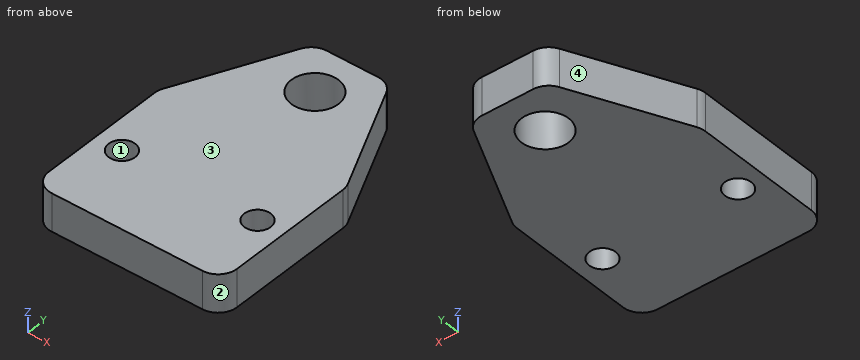
```python
from build123d import *

# Parameters (mm, degrees)
BOSS_EXTRU_1_DEPTH           = 10
ENL_V_MAT_EXTRU_1_DEPTH      = 77.870020164
ENL_V_MAT_EXTRU_1_DEPTH_BACK = 77.870020164
ESQUISSE2_R                  = 3.5
CONG_1_R                     = 5
ESQUISSE3_R                  = 6.25
ENL_V_MAT_EXTRU_2_DEPTH      = 77.870020164


with BuildPart() as part:
    # Esquisse1 → Boss.-Extru.1 (new body)
    with BuildSketch(Plane.XY):
        Polygon((-25, 0), (25, 0), (25, 40), (10, 72), (-10, 72), (-25, 40), align=None)
    extrude(amount=BOSS_EXTRU_1_DEPTH)

    # Esquisse2 → Enlèv. mat.-Extru.1 (cut, two sides: drawn at the far end of the back side and taken through both)
    with BuildSketch(Plane.XY.offset(10).offset(-ENL_V_MAT_EXTRU_1_DEPTH_BACK)):
        with Locations((18, 20)):
            Circle(ESQUISSE2_R)
        with Locations((-18, 20)):
            Circle(ESQUISSE2_R)
    extrude(amount=ENL_V_MAT_EXTRU_1_DEPTH + ENL_V_MAT_EXTRU_1_DEPTH_BACK, mode=Mode.SUBTRACT)

    # Congé1
    cong_1_edges = [part.edges().sort_by_distance(p)[0] for p in [
        (25, 0, 5),
        (-25, 0, 5),
        (-25, 40, 5),
        (-10, 72, 5),
        (10, 72, 5),
        (25, 40, 5),
    ]]
    fillet(cong_1_edges, radius=CONG_1_R)

    # Esquisse3 → Enlèv. mat.-Extru.2 (cut, through all)
    with BuildSketch(Plane.XY.offset(10)):
        with Locations((0, 60)):
            Circle(ESQUISSE3_R)
    extrude(amount=-ENL_V_MAT_EXTRU_2_DEPTH, mode=Mode.SUBTRACT)


solid = part.part
```
Geometry check sheet. Reference: the model listing, model coordinates, mm. Face numbers are marked on the shaded views. Give positions to 0.01 mm unless a question says otherwise; leave off trailing zeros. Order: outer loops, then holes, each group sorted by start corner. A loop starts at its lowest first (then second) coordinate and runs counter-clockwise, first axis right, second up. Notation, with made-up numbers: (-33, 24) -> (26, 24) arc R18 ccw to (26, 30) -> close; hole circle Ø4 at (34, -17.5). An arc over 180 degrees is marked (long way). Write each question's results on one line, items separated by ' | '. Start each with the question number.
(1) Mould release check, pull along X, two halves, no side actions. Record for the marked faces 1, 2, 3 and 4: pulls with the +X half, pulls with the -X half, needs draft (parallel to the pull), parting line crosses it, or undercut.
(2) Scan lines: line 1 (X direction, y = 20, z = 5.5); line 2 (Y direction, x = 0, z = 3); line 3 (X direction, y = 22, z = 9.5). Record each from-to range of solid material in increasing order.
(3) Sectioned sample at D-D (y = 57.5). Enter the section's corners in (x, z), plus the area to 3 significant figures.
(4) Sectioned sample at C-C (x = -18). Enter the section's corners in (y, z).
(5) Sectioned sample at A-A (y = 20). Enter the section's corners in (x, z), plus the area to 3 significant figures.
(6) Sectioned sample at B-B (z = 4). Enter the section's corners in (x, y), plus the area to 3 significant figures.
Answer below:
1) face 1: undercut | face 2: pulls with the +X half | face 3: needs draft | face 4: pulls with the -X half
2) line 1: -25 to -21.5, -14.5 to 14.5, 21.5 to 25 | line 2: 0 to 53.75, 66.25 to 72 | line 3: -25 to -20.87, -15.13 to 15.13, 20.87 to 25
3) outline: (-16.8, 0) -> (-5.73, 0) -> (-5.73, 10) -> (-16.8, 10) -> close; (5.73, 0) -> (16.8, 0) -> (16.8, 10) -> (5.73, 10) -> close | area: 221 mm2
4) outline: (0, 0) -> (16.5, 0) -> (16.5, 10) -> (0, 10) -> close; (23.5, 0) -> (54.93, 0) -> (54.93, 10) -> (23.5, 10) -> close
5) outline: (-25, 0) -> (-21.5, 0) -> (-21.5, 10) -> (-25, 10) -> close; (-14.5, 0) -> (14.5, 0) -> (14.5, 10) -> (-14.5, 10) -> close; (21.5, 0) -> (25, 0) -> (25, 10) -> (21.5, 10) -> close | area: 360 mm2
6) outline: (-25, 5) arc R5 ccw to (-20, 0) -> (20, 0) arc R5 ccw to (25, 5) -> (25, 38.89) arc R5 ccw to (24.53, 41.01) -> (11.35, 69.12) arc R5 ccw to (6.82, 72) -> (-6.82, 72) arc R5 ccw to (-11.35, 69.12) -> (-24.53, 41.01) arc R5 ccw to (-25, 38.89) -> close; hole circle Ø7 at (-18, 20); hole circle Ø12.5 at (0, 60); hole circle Ø7 at (18, 20) | area: 2,910 mm2
